Could you check a few things on this model? Use its own coordinates, in mm. A direction names the side the tool comes from. Coordinates: 2 decimals unless noted, no trailing zeros. Order: outer loops, then holes, each group sorted by start corner. A loop starts at its lowest first (then second) coordinate and runs counter-clockwise, first axis right, second up. Notation, with made-up numbers: (53, 12.5) - (93, 12.5) arc R14 ccw to (93, 23.5) - close; hole circle Ø2 at (58.5, -10). An arc over 180 degrees is marked (long way). One line per item, written item: value. Start each with the question number.
from build123d import *

# Parameters (mm, degrees)
EXTRUDE_1_DEPTH      = 13.7
EXTRUDE_2_DEPTH      = 9.7
SKETCH_3_W           = 11.5
SKETCH_3_H           = 22.7
EXTRUDE_3_DEPTH      = 13.7
SKETCH_4_W           = 11.5
SKETCH_4_H           = 2.8
EXTRUDE_4_DEPTH      = 2.4
SKETCH_5_W           = 11.5
SKETCH_5_H           = 2.8
EXTRUDE_5_DEPTH      = 2.4
SKETCH_6_W           = 9.748758204
SKETCH_6_H           = 1.713624198
CUT_EXTRUDE_7_DEPTH  = 2.8
SKETCH_7_W           = 9.748758204
SKETCH_7_H           = 1.35
EXTRUDE_8_DEPTH      = 4
CHAMFER_1_SIZE       = 1.2
SKETCH_8_R           = 2.5
EXTRUDE_9_DEPTH      = 0.25
SKETCH_9_R           = 1.25
CUT_EXTRUDE_10_DEPTH = 39.014240753


with BuildPart() as part:
    # Эскиз1 → Вытянуть1 (new body)
    with BuildSketch(Plane(origin=(0, 0, 0), x_dir=(1, 0, 0), z_dir=(0, 1, 0))):
        with BuildLine():
            Line((-13.25, 10), (13.25, 10))
            Line((13.25, 10), (13.25, -10))
            Line((13.25, -10), (-13.25, -10))
            ThreePointArc((-13.25, -10), (-23.25, 0), (-13.25, 10))
        make_face()
    extrude(amount=EXTRUDE_1_DEPTH)

    # Эскиз2 → Вытянуть2 (add)
    with BuildSketch(Plane(origin=(0, 13.7, 0), x_dir=(1, 0, 0), z_dir=(0, 1, 0))):
        with BuildLine():
            Line((-14.368033989, 1), (-12.131966011, 1))
            ThreePointArc((-12.131966011, 1), (-13.25, -1.5), (-14.368033989, 1))
        make_face()
    extrude(amount=EXTRUDE_2_DEPTH)

    # Эскиз3 → Вытянуть3 (add)
    with BuildSketch(Plane.XZ):
        with Locations((7.5, 0)):
            Rectangle(SKETCH_3_W, SKETCH_3_H)
    extrude(amount=EXTRUDE_3_DEPTH)

    # Эскиз4 → Вытянуть4 (add)
    with BuildSketch(Plane(origin=(0, 0, -10), x_dir=(-1, 0, 0), z_dir=(0, 0, -1))):
        with Locations((-7.5, 1.4)):
            Rectangle(SKETCH_4_W, SKETCH_4_H)
    extrude(amount=EXTRUDE_4_DEPTH)

    # Эскиз5 → Вытянуть5 (add)
    with BuildSketch(Plane.XY.offset(10)):
        with Locations((7.5, 1.4)):
            Rectangle(SKETCH_5_W, SKETCH_5_H)
    extrude(amount=EXTRUDE_5_DEPTH)

    # Эскиз6 → Вытянуть7 (cut)
    with BuildSketch(Plane(origin=(0, 2.8, 0), x_dir=(1, 0, 0), z_dir=(0, 1, 0))):
        with Locations((7.563806599, 10.856812099)):
            Rectangle(SKETCH_6_W, SKETCH_6_H)
        with Locations((7.563806599, -10.856812099)):
            Rectangle(SKETCH_6_W, SKETCH_6_H)
    extrude(amount=-CUT_EXTRUDE_7_DEPTH, mode=Mode.SUBTRACT)

    # Эскиз7 → Вытянуть8 (add)
    with BuildSketch(Plane(origin=(0, 0, 0), x_dir=(1, 0, 0), z_dir=(0, 1, 0))):
        with Locations((7.563806599, 10.675)):
            Rectangle(SKETCH_7_W, SKETCH_7_H)
        with Locations((7.563806599, -10.675)):
            Rectangle(SKETCH_7_W, SKETCH_7_H)
    extrude(amount=EXTRUDE_8_DEPTH)

    # Фаска1
    chamfer_1_edges = [part.edges().sort_by_distance(p)[0] for p in [
        (7.563806599, 4, -11.35),
        (7.563806599, 4, 11.35),
    ]]
    chamfer(chamfer_1_edges, length=CHAMFER_1_SIZE)

    # Эскиз8 → Вытянуть9 (add)
    with BuildSketch(Plane(origin=(0, 13.7, 0), x_dir=(1, 0, 0), z_dir=(0, 1, 0))):
        with Locations(Location((-13.25, 0, 0), (0, 0, 90))):
            Circle(SKETCH_8_R)
    extrude(amount=EXTRUDE_9_DEPTH)

    # Эскиз9 → Вытянуть10 (cut, through all)
    with BuildSketch(Plane(origin=(0, 13.7, 0), x_dir=(1, 0, 0), z_dir=(0, 1, 0))):
        with Locations(Location((-6.25, -8, 0), (0, 0, 270))):
            Circle(SKETCH_9_R)
    extrude(amount=-CUT_EXTRUDE_10_DEPTH, mode=Mode.SUBTRACT)


solid = part.part
Q1. If I drill on L1, parallel to Y at x = -13.5, z = -3.5; L2, parallel to Y at x = 7, z = -0.5; L3, parallel to X at y = 6.5, z = 8, over which ranges is the centre line in solid material (lowest first)?
Q2. I want a section at A-A on x = -6.25. Please give me the cut outline in (y, z).
Q3. We'd pull the mould along Z, two halves only. Please class faces 1 (the flat face through (8, 0, -12)), 2 (the flat face through (7, -5, 11.35)), 3 (the flat face through (8, 1, -12.4)): +Z half, -Z half, draft (parallel to the pull), parting line (faces both ways), or undercut.
Q4. I want a section at B-B on z = 8. Please give me the cut outline in (x, y), then the cut area to 3 significant figures.
Q5. I want a section at D-D on x = 9. Please give me the cut outline in (y, z).
Q6. I want a section at C-C on y = 12.5. Please give me the cut outline in (x, z).
Q7. I'm going to push flat-ended pins straight in: pin 1 (2.5 mm diameter, centred on x = 6, z = -11.5, fed in from +Y); pin 2 (5 mm diameter, centred on x = 0, z = 6.5, fed in from +Y); pin 3 (1.1 mm diameter, centred on x = -13.5, y = 16.5, fed in from -Z). Where does each tip first touch, or does it pass through?
Q8. Which directions (+Z, -Z, +X, -X, +Y, -Y) give clear straight access to the entire face, cutting with the end or side of a thin tool? Please do faces 4 (the cylindrical face through (-13.2, 18.6, 1.5)), 5 (the flat face through (7, 1, 11.714)), 6 (the flat face through (12.438, 3.3, -10.5)), 7 (the flat face through (7, 0, 12)).
Values follow:
1. L1: y = 0 to 13.7
1. L2: y = -13.7 to 13.7
1. L3: x = -19.25 to -7.5, -5 to 13.25
2. outline: (0, -10) - (13.7, -10) - (13.7, 6.75) - (0, 6.75) - close; (0, 9.25) - (13.7, 9.25) - (13.7, 10) - (0, 10) - close
3. face 1: draft
3. face 2: undercut
3. face 3: -Z half
4. outline: (-19.25, 0) - (-7.5, 0) - (-7.5, 13.7) - (-19.25, 13.7) - close; (-5, 0) - (1.75, 0) - (1.75, -13.7) - (13.25, -13.7) - (13.25, 13.7) - (-5, 13.7) - close
4. area: 569 mm^2
5. outline: (-13.7, -11.35) - (2.8, -11.35) - (4, -10.15) - (4, -10) - (13.7, -10) - (13.7, 10) - (4, 10) - (4, 10.15) - (2.8, 11.35) - (-13.7, 11.35) - close; (0, -12.4) - (2.8, -12.4) - (2.8, -11.71) - (0, -11.71) - close; (0, 11.71) - (2.8, 11.71) - (2.8, 12.4) - (0, 12.4) - close
6. outline: (-13.25, -10) - (13.25, -10) - (13.25, 10) - (-13.25, 10) arc R10 ccw to start; hole circle Ø2.5 at (-6.25, 8)
7. pin 1: stops at y = 3.9
7. pin 2: stops at y = 13.7
7. pin 3: stops at z = -1
8. face 4: +Y
8. face 5: +Y, -Y
8. face 6: -Z, +X, +Y
8. face 7: +Z, +X, -X, -Y
